```python
from build123d import *

# Parameters (mm, degrees)
SKETCH1_W           = 20
SKETCH1_H           = 20
SKETCH1_R           = 7.5
BOSS_EXTRUDE1_DEPTH = 60
SKETCH2_R           = 1.15
CUT_EXTRUDE1_DEPTH  = 21


with BuildPart() as part:
    # Sketch1 → Boss-Extrude1 (new body)
    with BuildSketch(Plane.XY):
        with Locations((10, 10)):
            Rectangle(SKETCH1_W, SKETCH1_H)
        with Locations((10, 10)):
            Circle(SKETCH1_R, mode=Mode.SUBTRACT)
    extrude(amount=BOSS_EXTRUDE1_DEPTH)

    # Sketch2 → Cut-Extrude1 (cut, through all)
    with BuildSketch(Plane(origin=(0, 20, 0), x_dir=(1, 0, 0), z_dir=(0, 1, 0))):
        with Locations((3, -57)):
            Circle(SKETCH2_R)
        with Locations((17, -57)):
            Circle(SKETCH2_R)
        with Locations((3, -3)):
            Circle(SKETCH2_R)
        with Locations((17, -3)):
            Circle(SKETCH2_R)
    extrude(amount=-CUT_EXTRUDE1_DEPTH, mode=Mode.SUBTRACT)


solid = part.part
```
For this review, take the finished solid that the model builds, in its own axes (mm). Coordinates: 2 decimals unless noted, no trailing zeros. Order: outer loops, then holes, each group sorted by start corner. A loop starts at its lowest first (then second) coordinate and runs counter-clockwise, first axis right, second up. Notation, with made-up numbers: (75.25, -24) -> (96.25, -24) arc R12 ccw to (96.25, -2) -> close; hole circle Ø2 at (-33.75, -2). An arc over 180 degrees is marked (long way). Use CSV: the item, a comma, the result in double quotes. Start each with the question number.
Item 1: Insertion check: pin 1 (12 mm diameter, centred on x = 16.5, y = 13, fed in from +Z); pin 2 (2 mm diameter, centred on x = 3, z = 3, fed in from -Y). Each pin has a flat end and moves straight along its axis. Give the tip position at first contact, or say it passes through.
Item 2: Draft analysis for pull direction X (two halves, no side actions). For faces 1 (the face through (10, 0, 30)), 2 (the face through (4.5, 15.1, 29.6)), 3 (the face through (18.097, 10.14, 2.655)), 4 (the face through (20, 10, 30)), state which applies: pulls with the +X half, pulls with the -X half, needs draft (parallel to the pull), parting line crosses it, or undercut.
Item 3: We need section D-D, the plane y = 15.75. Give the boundary of the cut face in (x, z), then the cut area to 3 significant figures.
Item 4: We need section C-C, the plane y = 9. Give the boundary of the cut face in (x, z), then the cut area to 3 significant figures.
Item 5: Wall thickness on probe 1 along Z at (x, y) = (17, 14.25); probe 2 along X at (y, z) = (12, 57); probe 3 along Y at (x, z) = (10, 13.5): over which ranges is each line inside the solid? List them lowest first.
Item 6: We need section A-A, the plane x = 10. Give the boundary of the cut face in (y, z), then the cut area to 3 significant figures.
Item 7: We need section B-B, the plane z = 13. Give the boundary of the cut face in (x, y), then the cut area to 3 significant figures.
Derived:
1,pin 1,"stops at z = 60"
1,pin 2,"passes through"
2,face 1,"needs draft"
2,face 2,"undercut"
2,face 3,"undercut"
2,face 4,"pulls with the +X half"
3,outline,"(0, 0) -> (5.18, 0) -> (5.18, 60) -> (0, 60) -> close; (14.82, 0) -> (20, 0) -> (20, 60) -> (14.82, 60) -> close; hole circle Ø2.3 at (3, 3); hole circle Ø2.3 at (3, 57); hole circle Ø2.3 at (17, 3); hole circle Ø2.3 at (17, 57)"
3,area,"606 mm^2"
4,outline,"(0, 0) -> (2.57, 0) -> (2.57, 1.93) arc R1.15 cw to (2.57, 4.07) -> (2.57, 55.93) arc R1.15 cw to (2.57, 58.07) -> (2.57, 60) -> (0, 60) -> close; (17.43, 0) -> (20, 0) -> (20, 60) -> (17.43, 60) -> (17.43, 58.07) arc R1.15 cw to (17.43, 55.93) -> (17.43, 4.07) arc R1.15 cw to (17.43, 1.93) -> close"
4,area,"304 mm^2"
5,probe 1,"z = 0 to 1.85, 4.15 to 55.85, 58.15 to 60"
5,probe 2,"x = 0 to 1.85, 18.15 to 20"
5,probe 3,"y = 0 to 2.5, 17.5 to 20"
6,outline,"(0, 0) -> (2.5, 0) -> (2.5, 60) -> (0, 60) -> close; (17.5, 0) -> (20, 0) -> (20, 60) -> (17.5, 60) -> close"
6,area,"300 mm^2"
7,outline,"(0, 0) -> (20, 0) -> (20, 20) -> (0, 20) -> close; hole circle Ø15 at (10, 10)"
7,area,"223 mm^2"
